Verification items for the finished model (mm, model axes). Round coordinates to 2 decimals unless told otherwise and drop trailing zeros. Write each loop counter-clockwise with the first axis right and the second up, starting at its lowest first coordinate (ties: lowest second). Pieces come first, ordered by that corner, then holes.
from build123d import *

# Parameters (mm, degrees)
F1_DEPTH = 19
F3_DEPTH = 8


with BuildPart() as f1:
    # F0 (on Front) → F1 (new body)
    with BuildSketch(Plane.XZ):
        with BuildLine():
            ThreePointArc((-175, 190), (-266.991847, 149.807266), (-300, 55))
            Line((-300, 55), (-300, 0))
            Line((-300, 0), (0, 0))
            Line((0, 0), (0, 190))
            Line((0, 190), (-175, 190))
        make_face()
    extrude(amount=F1_DEPTH)

    # F2 (on face) → F3 (cut)
    with BuildSketch(Plane.XZ.offset(19)):
        with BuildLine():
            Line((0, 171), (0, 179))
            Line((0, 179), (-175, 179))
            ThreePointArc((-175, 179), (-254.798891, 137.960271), (-289, 55))
            Line((-289, 55), (-289, 0))
            Line((-289, 0), (-281, 0))
            Line((-281, 0), (-281, 55))
            ThreePointArc((-281, 55), (-247.509978, 130.828083), (-175, 171))
            Line((-175, 171), (0, 171))
        make_face()
    extrude(amount=-F3_DEPTH, mode=Mode.SUBTRACT)


solid = f1.part
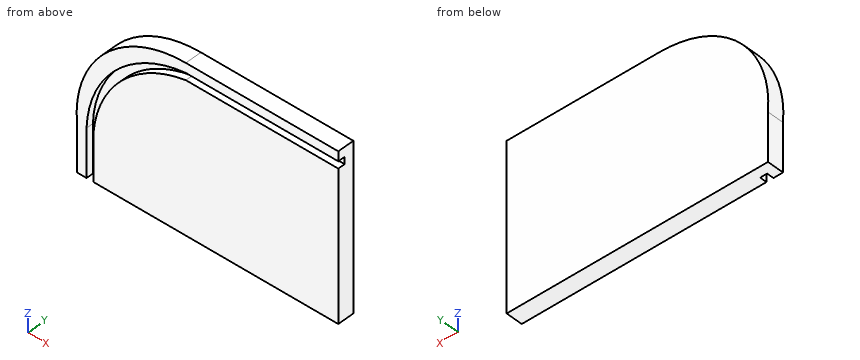
Q1. Sectioned sample at A-A (x = -147.5). Enter the section's corners in (y, z).
Recorded:
outline: (-19, 0) - (0, 0) - (0, 190) - (-19, 190) - (-19, 179) - (-11, 179) - (-11, 171) - (-19, 171) - close
Q2. Sectioned sample at D-D (z = 175). Enter the section's corners in (x, y), plus the area to 3 significant figures.
Recorded:
outline: (-234.47, -19) - (-194.72, -19) - (-194.72, -11) - (0, -11) - (0, 0) - (-234.47, 0) - close
area: 2,900 mm2
Q3. Depth check by flat-ended pin: P1, Ø2.5, axis at y = -13.5, z = 31.5, coming from the -X side. Enter the tip coordinate at first touch or a pass-through.
Recorded:
P1: stops at x = -300
Q4. Sectioned sample at B-B (y = -7.5). Enter the section's corners in (x, z), plus the area to 3 significant figures.
Recorded:
outline: (-300, 0) - (0, 0) - (0, 190) - (-175, 190) arc R125.37 ccw to (-300, 55) - close
area: 53,700 mm2
Q5. Material ranges on line 1 along Z through (x, y) = (-148.5, -11.5); line 2 along Y through (x, z) = (-260, 118); line 3 along Z through (x, y) = (-262.5, -17), recorded low to high.
Recorded:
line 1: z = 0 to 171, 179 to 190
line 2: y = -11 to 0
line 3: z = 0 to 110.87, 128.77 to 154.42
Q6. Sectioned sample at C-C (z = 103). Enter the section's corners in (x, y).
Recorded:
outline: (-294.35, -19) - (-277.79, -19) - (-277.79, -11) - (-266.94, -11) - (-266.94, -19) - (0, -19) - (0, 0) - (-294.35, 0) - close
